from build123d import *

# Parameters (mm, degrees)
F0_R     = 11
F1_DEPTH = 7


with BuildPart() as f1:
    # F0 (on Top) → F1 (new body)
    with BuildSketch(Plane.XY):
        with BuildLine():
            ThreePointArc((-10.281257, 34.502407), (-13.176009, 29.732102), (-13.977698, 24.210082))
            ThreePointArc((-13.977698, 24.210082), (-24.891005, 26.119838), (-33.774991, 19.5))
            ThreePointArc((-33.774991, 19.5), (-35.564126, 14.053951), (-35.02059, 8.347374))
            ThreePointArc((-35.02059, 8.347374), (-32.33676, 3.455292), (-27.955395, 0))
            ThreePointArc((-27.955395, 0), (-35.065946, -8.496324), (-33.774991, -19.5))
            ThreePointArc((-33.774991, -19.5), (-29.953142, -23.772461), (-24.739333, -26.155034))
            ThreePointArc((-24.739333, -26.155034), (-19.160751, -26.276809), (-13.977698, -24.210082))
            ThreePointArc((-13.977698, -24.210082), (-10.174941, -34.616162), (0, -39))
            ThreePointArc((0, -39), (5.610985, -37.826412), (10.281257, -34.502407))
            ThreePointArc((10.281257, -34.502407), (13.176009, -29.732102), (13.977698, -24.210082))
            ThreePointArc((13.977698, -24.210082), (24.891005, -26.119838), (33.774991, -19.5))
            ThreePointArc((33.774991, -19.5), (35.564126, -14.053951), (35.02059, -8.347374))
            ThreePointArc((35.02059, -8.347374), (32.33676, -3.455292), (27.955395, 0))
            ThreePointArc((27.955395, 0), (35.065946, 8.496324), (33.774991, 19.5))
            ThreePointArc((33.774991, 19.5), (29.953142, 23.772461), (24.739333, 26.155034))
            ThreePointArc((24.739333, 26.155034), (19.160751, 26.276809), (13.977698, 24.210082))
            ThreePointArc((13.977698, 24.210082), (10.174941, 34.616162), (0, 39))
            ThreePointArc((0, 39), (-5.610985, 37.826412), (-10.281257, 34.502407))
        make_face()
        with Locations((-21.650635, -12.5)):
            Circle(F0_R, mode=Mode.SUBTRACT)
        with BuildLine():
            ThreePointArc((-6.30476, -12.5), (-7, -12.875644), (-7.672937, -13.289918))
            ThreePointArc((-7.672937, -13.289918), (-7.650635, -12.5), (-7.672937, -11.710082))
            ThreePointArc((-7.672937, -11.710082), (-7, -12.124356), (-6.30476, -12.5))
        make_face(mode=Mode.SUBTRACT)
        with Locations((0, -25)):
            Circle(F0_R, mode=Mode.SUBTRACT)
        with BuildLine():
            ThreePointArc((7.672937, -11.710082), (7.650635, -12.5), (7.672937, -13.289918))
            ThreePointArc((7.672937, -13.289918), (7, -12.875644), (6.30476, -12.5))
            ThreePointArc((6.30476, -12.5), (7, -12.124356), (7.672937, -11.710082))
        make_face(mode=Mode.SUBTRACT)
        with Locations((21.650635, -12.5)):
            Circle(F0_R, mode=Mode.SUBTRACT)
        with Locations((-21.650635, 12.5)):
            Circle(F0_R, mode=Mode.SUBTRACT)
        with BuildLine():
            ThreePointArc((-15.345875, 0), (-14.650635, 0.375644), (-13.977698, 0.789918))
            ThreePointArc((-13.977698, 0.789918), (-14, 0), (-13.977698, -0.789918))
            ThreePointArc((-13.977698, -0.789918), (-14.650635, -0.375644), (-15.345875, 0))
        make_face(mode=Mode.SUBTRACT)
        with BuildLine():
            ThreePointArc((-7.672937, 11.710082), (-7.650635, 12.5), (-7.672937, 13.289918))
            ThreePointArc((-7.672937, 13.289918), (-7, 12.875644), (-6.30476, 12.5))
            ThreePointArc((-6.30476, 12.5), (-7, 12.124356), (-7.672937, 11.710082))
        make_face(mode=Mode.SUBTRACT)
        Circle(F0_R, mode=Mode.SUBTRACT)
        with BuildLine():
            ThreePointArc((13.977698, -0.789918), (14, 0), (13.977698, 0.789918))
            ThreePointArc((13.977698, 0.789918), (14.650635, 0.375644), (15.345875, 0))
            ThreePointArc((15.345875, 0), (14.650635, -0.375644), (13.977698, -0.789918))
        make_face(mode=Mode.SUBTRACT)
        with BuildLine():
            ThreePointArc((6.30476, 12.5), (7, 12.875644), (7.672937, 13.289918))
            ThreePointArc((7.672937, 13.289918), (7.650635, 12.5), (7.672937, 11.710082))
            ThreePointArc((7.672937, 11.710082), (7, 12.124356), (6.30476, 12.5))
        make_face(mode=Mode.SUBTRACT)
        with Locations((21.650635, 12.5)):
            Circle(F0_R, mode=Mode.SUBTRACT)
        with Locations((0, 25)):
            Circle(F0_R, mode=Mode.SUBTRACT)
        with BuildLine():
            ThreePointArc((-35.02059, 8.347374), (-35.564126, 14.053951), (-33.774991, 19.5))
            ThreePointArc((-33.774991, 19.5), (-36.303554, 14.098273), (-37.869486, 8.343263))
            ThreePointArc((-37.869486, 8.343263), (-36.4456, 8.734654), (-35.02059, 8.347374))
        make_face()
        with BuildLine():
            ThreePointArc((-11.709265, 36.967568), (-10.658367, 35.930142), (-10.281257, 34.502407))
            ThreePointArc((-10.281257, 34.502407), (-5.610985, 37.826412), (0, 39))
            ThreePointArc((0, 39), (-5.942314, 38.488936), (-11.709265, 36.967568))
        make_face()
        with BuildLine():
            ThreePointArc((-24.739333, -26.155034), (-29.953142, -23.772461), (-33.774991, -19.5))
            ThreePointArc((-33.774991, -19.5), (-30.36124, -24.390663), (-26.16022, -28.624305))
            ThreePointArc((-26.16022, -28.624305), (-25.787232, -27.195488), (-24.739333, -26.155034))
        make_face()
        with BuildLine():
            ThreePointArc((26.16022, 28.624305), (25.787232, 27.195488), (24.739333, 26.155034))
            ThreePointArc((24.739333, 26.155034), (29.953142, 23.772461), (33.774991, 19.5))
            ThreePointArc((33.774991, 19.5), (30.36124, 24.390663), (26.16022, 28.624305))
        make_face()
        with BuildLine():
            ThreePointArc((10.281257, -34.502407), (5.610985, -37.826412), (0, -39))
            ThreePointArc((0, -39), (5.942314, -38.488936), (11.709265, -36.967568))
            ThreePointArc((11.709265, -36.967568), (10.658367, -35.930142), (10.281257, -34.502407))
        make_face()
        with BuildLine():
            ThreePointArc((37.869486, -8.343263), (36.4456, -8.734654), (35.02059, -8.347374))
            ThreePointArc((35.02059, -8.347374), (35.564126, -14.053951), (33.774991, -19.5))
            ThreePointArc((33.774991, -19.5), (36.303554, -14.098273), (37.869486, -8.343263))
        make_face()
    extrude(amount=F1_DEPTH)


solid = f1.part
Geometry check sheet. Reference: the model listing, model coordinates, mm. Round coordinates to 2 decimals unless told otherwise and drop trailing zeros. Order: outer loops, then holes, each group sorted by start corner. A loop starts at its lowest first (then second) coordinate and runs counter-clockwise, first axis right, second up. Notation, with made-up numbers: M -28.75,58 L -22.75,58 A9 ccw -22.75,75 Z; hole C -27.75,-0.75 d4. An arc over 180 degrees is marked long. Write each question's results on one line, items separated by ' | '. Start each with the question number.
1. Draft check along X on faces 1 (the face through (13.149, -29.806, 3.451)), 2 (the face through (-2.38, -35.74, 3.45)), 3 (the face through (36.275, -14.177, 3.451)), 4 (the face through (-30.41, -24.33, 3.45)). Enter one of: pulls with the +X half, pulls with the -X half, needs draft (parallel to the pull), parting line crosses it, or undercut.
2. Cross-section at B-B on y = -21.5. Record the boundary of the cut face in (x, z).
3. Go/stop test with flat-tipped pins: P1, Ø1.5, axis at y = 30.5, z = 3, coming from the -X side; P2, Ø1.5, axis at y = -1, z = 1, coming from the +X side; P3, Ø4, axis at y = -1.5, z = 1, coming from the -X side; P4, Ø20, axis at x = -21.65, y = 12.5, coming from the +Z side. Record where each tip stops, or that it passes through.
4. Cross-section at C-C on x = -23. Record the boundary of the cut face in (y, z).
5. Cross-section at D-D on z = 6. Give the number of separate pieces and of enclosed holes in the cut face, plus the area to 3 significant figures.
6. Cross-section at A-A on x = -3. Record the boundary of the cut face in (y, z), plus the area to 3 significant figures.
7. Material ranges on L1, parallel to Y at x = -22, z = 3.5; L2, parallel to Y at x = 16, z = 6; L3, parallel to X at y = 15.5, z = 3.5, recorded low to high. Write a range as from..to.
Resolved:
1) face 1: undercut | face 2: undercut | face 3: pulls with the +X half | face 4: pulls with the -X half
2) outline: M -32.53,0 L -27.98,0 L -27.98,7 L -32.53,7 Z; M -15.33,0 L -10.43,0 L -10.43,7 L -15.33,7 Z; M 10.43,0 L 15.33,0 L 15.33,7 L 10.43,7 Z; M 27.98,0 L 32.37,0 L 32.37,7 L 27.98,7 Z
3) P1: x = -13.17 | P2: x = 30.62 | P3: x = -32.37 | P4: through
4) outline: M -26.43,0 L -23.42,0 L -23.42,7 L -26.43,7 Z; M -1.58,0 L 1.58,0 L 1.58,7 L -1.58,7 Z; M 23.42,0 L 26.43,0 L 26.43,7 L 23.42,7 Z
5) separate pieces: 1 | enclosed holes: 13 | area: 1,410 mm2
6) outline: M -38.67,0 L -35.58,0 L -35.58,7 L -38.67,7 Z; M -14.42,0 L -10.58,0 L -10.58,7 L -14.42,7 Z; M 10.58,0 L 14.42,0 L 14.42,7 L 10.58,7 Z; M 35.58,0 L 38.87,0 L 38.87,7 L 35.58,7 Z | area: 98.3 mm2
7) L1: -26.5..-23.49, -1.51..1.51, 23.49..26.5 | L2: -25.31..-21.94, -3.06..3.06, 21.94..25.31 | L3: -35.75..-32.23, -11.07..-5.55, 5.55..11.07, 32.23..35.33
